Work out the finished part from the listing and answer in its coordinate system (mm). Round coordinates to 2 decimals unless told otherwise and drop trailing zeros. Write each loop counter-clockwise with the first axis right and the second up, starting at its lowest first coordinate (ties: lowest second). Pieces come first, ordered by that corner, then holes. Notation, with made-up numbers: M -10.75,15.5 L 47.25,15.5 A8 cw 47.25,30.5 Z; hole C -10,-38 d4. An arc over 180 degrees is marked long. Answer in a Markdown table with one row per item.
```python
from build123d import *

# Parameters (mm, degrees)
SKETCH1_R             = 11.1125
SKETCH1_R_2           = 6.35
SKETCH1_R_3           = 4.7625
BOSS_EXTRUDE1_DEPTH   = 3.175
M3X0_5_TAPPED_HOLE1_D = 2.5


with BuildPart() as part:
    # Sketch1 → Boss-Extrude1 (new, symmetric)
    with BuildSketch(Plane(origin=(0, 0, 0), x_dir=(0, 0, -1), z_dir=(1, 0, 0))):
        with BuildLine():
            ThreePointArc((109.135384069, 42.254910239), (105.621138378, 44.242227481), (101.584158555, 44.195897144))
            Line((101.584158555, 44.195897144), (-4.066677309, 14.438217884))
            ThreePointArc((-4.066677309, 14.438217884), (-14.858890744, -2.052648501), (0, -15))
            Line((0, -15), (106.075609583, -29.237803609))
            ThreePointArc((106.075609583, -29.237803609), (136.491140548, -12.979579055), (130.699290202, 21.018786481))
            Line((130.699290202, 21.018786481), (109.135384069, 42.254910239))
        make_face()
        Circle(SKETCH1_R, mode=Mode.SUBTRACT)
        with Locations((110, 0)):
            Circle(SKETCH1_R_2, mode=Mode.SUBTRACT)
        with Locations((103.688664063, 36.724119389)):
            Circle(SKETCH1_R_3, mode=Mode.SUBTRACT)
    extrude(amount=BOSS_EXTRUDE1_DEPTH, both=True)

    # M3x0.5 Tapped Hole1 (through all)
    with Locations(Plane(origin=(3.175, 0, 0), x_dir=(0, 0, -1), z_dir=(1, 0, 0))):
        with Locations((123.200861683, 18.852784299), (110, 0), (96.799138317, -18.852784299)):
            Hole(M3X0_5_TAPPED_HOLE1_D / 2)


solid = part.part
```
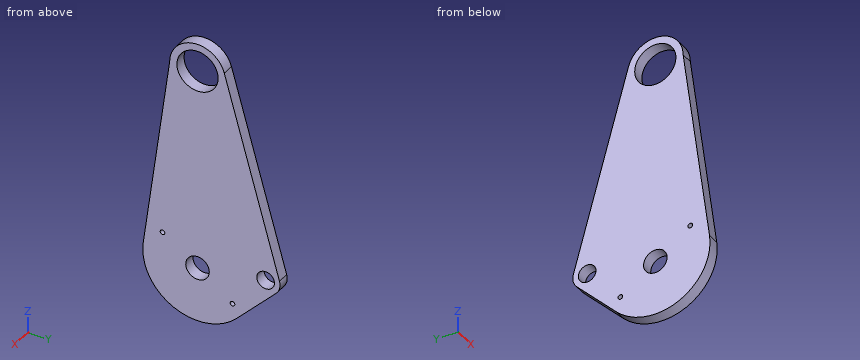
1. The part is cut by section C-C (z = 5.5). Determine the outline of the cut face in (x, y) (3 decimals), plus the area to 3 significant figures.
Calculated:
| item | result |
|---|---|
| outline | M -3.175,-13.955 L 3.175,-13.955 L 3.175,-9.656 L -3.175,-9.656 Z; M -3.175,9.656 L 3.175,9.656 L 3.175,13.955 L -3.175,13.955 Z |
| area | 54.6 mm² |
2. Given pin 1 (3 mm diameter, centred on x = 0.5, y = 22.5, fed in from -Z), flat-ended and moving along its own axis, determine where the tip first touches the part or whether it passes through.
Calculated:
| item | result |
|---|---|
| pin 1 | stops at z = -130.72 |
3. The part is cut by section A-A (y = 0). Count the separate pieces of the cut face and the enclosed holes in it, plus the area to 3 significant figures.
Calculated:
| item | result |
|---|---|
| separate pieces | 3 |
| enclosed holes | 0 |
| area | 759 mm² |
4. Consider line 1 along Y through (x, z) = (0.75, -110); line 2 along Y through (x, z) = (-1, -4); line 3 along Z through (x, y) = (-0.5, -1.5). Determine where each line is inside the solid, lowest interval first. Write a range as from..to.
Calculated:
| item | result |
|---|---|
| line 1 | y = -29.5..-6.35, 6.35..41.4 |
| line 2 | y = -15.54..-10.37, 10.37..16.71 |
| line 3 | z = -139.46..-116.17, -103.83..-11.01, 11.01..14.92 |
5. The part is cut by section D-D (z = -49.5). Determine the outline of the cut face in (x, y) (3 decimals).
Calculated:
| item | result |
|---|---|
| outline | M -3.175,-21.644 L 3.175,-21.644 L 3.175,29.526 L -3.175,29.526 Z |
